Autodesk Inventor part; units mm, degrees
ref_plane "YZ Plane" through (0, 0, 0) normal (1, 0, 0) x (0, 1, 0)
ref_plane "XZ Plane" through (0, 0, 0) normal (0, 1, 0) x (-1, 0, 0)
ref_plane "XY Plane" through (0, 0, 0) normal (0, 0, 1) x (1, 0, 0)
sketch "Эскиз1" plane through (0, 0, 0) normal (0, 0, 1) x (1, 0, 0)
  circle A0 centre (0, 0) radius 13
  circle A1 centre (0, 9) radius 1.5
  circle A2 centre (-9, 0) radius 1.5
  circle A3 centre (0, -9) radius 1.5
  circle A4 centre (9, 0) radius 1.5
  dimension "d0" = 26
  dimension "d1" = 3
  dimension "d2" = 9
  dimension "d5" = 360
extrude "Выдавливание1" add sketch "Эскиз1" along normal blind 7
sketch "Эскиз2" plane through (0, 0, 7) normal (0, 0, 1) x (1, 0, 0)
  circle A0 centre (0, 0) radius 13
  circle A1 centre (9, 0) radius 1.5
  circle A2 centre (0, -9) radius 1.5
  circle A3 centre (-9, 0) radius 1.5
  circle A4 centre (0, 9) radius 1.5
  circle A5 centre (0, 0) radius 9.5
  dimension "d9" = 19
extrude "Выдавливание2" add sketch "Эскиз2" along normal blind 5 contours A0 | A1 A5 | A5 A4 | A2 A5 | A5 A3 picked at (9.8174, -0.2697) picked at (-0.0593, 9.8216) picked at (0.0593, -9.8216) picked at (-9.8216, 0.0593)
sketch "Эскиз3" plane through (0, 0, 7) normal (0, 0, 1) x (1, 0, 0)
  arc A0 (-1.4487, 9.3889) -> (-9.3889, 1.4487) centre (0, 0) ccw
  arc A1 (-9.3889, -1.4487) -> (-9.3889, 1.4487) centre (-9, 0) ccw
  arc A2 (-9.3889, -1.4487) -> (-1.4487, -9.3889) centre (0, 0) ccw
  arc A3 (1.4487, -9.3889) -> (-1.4487, -9.3889) centre (0, -9) ccw
  arc A4 (1.4487, -9.3889) -> (9.3889, -1.4487) centre (0, 0) ccw
  arc A5 (9.3889, 1.4487) -> (9.3889, -1.4487) centre (9, 0) ccw
  arc A6 (9.3889, 1.4487) -> (1.4487, 9.3889) centre (0, 0) ccw
  arc A7 (-1.4487, 9.3889) -> (1.4487, 9.3889) centre (0, 9) ccw
  arc A8 (1.4487, 9.3889) -> (-1.4487, 9.3889) centre (0, 0) ccw
  circle A9 centre (0, 0) radius 9.5
  arc A10 (9.3889, -1.4487) -> (9.3889, 1.4487) centre (0, 0) ccw
  arc A11 (1.4487, -9.3889) -> (9.3889, -1.4487) centre (0, 0) ccw
  arc A12 (-1.4487, -9.3889) -> (1.4487, -9.3889) centre (0, 0) ccw
  arc A13 (-9.3889, -1.4487) -> (-1.4487, -9.3889) centre (0, 0) ccw
  arc A14 (-9.3889, 1.4487) -> (-9.3889, -1.4487) centre (0, 0) ccw
  arc A15 (-1.4487, 9.3889) -> (-9.3889, 1.4487) centre (0, 0) ccw
  arc A16 (1.4487, 9.3889) -> (-1.4487, 9.3889) centre (0, 0) ccw
  arc A17 (9.3889, 1.4487) -> (1.4487, 9.3889) centre (0, 0) ccw
  point P0 (-1.4487, -9.3889)
  point P1 (1.4487, -9.3889)
  point P2 (9.3889, -1.4487)
  point P3 (9.3889, 1.4487)
  point P4 (-9.3889, 1.4487)
  point P5 (-9.3889, -1.4487)
extrude "Выдавливание3" add sketch "Эскиз3" against normal blind 0.1 contours A8 A7 | A1 A9 | A9 A5 | A3 A9
sketch "Эскиз4" plane through (0, 0, 12) normal (0, 0, 1) x (1, 0, 0)
  circle A0 centre (-16.4751, 0) radius 1.5
  circle A1 centre (0, 9) radius 1.5
  arc A2 (1.4487, -9.3889) -> (-1.4487, -9.3889) centre (0, -9) ccw
  line L0 (0, 9) -> (0, -9)
  circle A3 centre (16.4751, 0) radius 1.5
  line L1 (-19.9502, -2.5984) -> (-13, -2.5984)
  line L2 (-13, -2.5984) -> (-13, 2.5984)
  line L3 (-13, 2.5984) -> (-19.9502, 2.5984)
  line L4 (-19.9502, 2.5984) -> (-19.9502, -2.5984)
  line L5 (-19.9502, -2.5984) -> (-13, 2.5984) construction
  line L6 (-13, -2.5984) -> (-19.9502, 2.5984) construction
  line L7 (-13, 2.5984) -> (-11.6906, 2.5984)
  circle A4 centre (0, 0) radius 13
  circle A5 centre (0, 0) radius 9.5
  line L8 (-13, -2.5984) -> (-12.3453, -2.5984)
  circle A6 centre (16.4751, 0) radius 1.5
  line L9 (19.9502, -2.5984) -> (13, -2.5984)
  line L10 (13, -2.5984) -> (13, 2.5984)
  line L11 (13, 2.5984) -> (19.9502, 2.5984)
  line L12 (19.9502, 2.5984) -> (19.9502, -2.5984)
  line L13 (19.9502, -2.5984) -> (13, 2.5984) construction
  line L14 (13, -2.5984) -> (19.9502, 2.5984) construction
  line L15 (13, 2.5984) -> (11.6906, 2.5984)
  line L16 (13, -2.5984) -> (12.3453, -2.5984)
  point P0 (12.7377, 2.5984)
  point P1 (12.7377, -2.5984)
  point P2 (-12.7377, -2.5984)
  point P3 (-12.7377, 2.5984)
  dimension "d14" = 3
extrude "Выдавливание4" add sketch "Эскиз4" against normal blind 3 contours L4 L3 L2 L1 | L2 A4 L8 | L2 L7 A4 | A4 L10 L16 | L15 L10 A4 | L10 L11 L12 L9
properties part number "вт2"
Can you work these out from the model? Positions are in its coordinate system, mm. A direction names the side the tool comes from. Coordinates: 2 decimals unless noted, no trailing zeros. Write each loop counter-clockwise with the first axis right and the second up, starting at its lowest first coordinate (ties: lowest second). Pieces come first, ordered by that corner, then holes. Notation, with made-up numbers: M -8,67 L 3,67 A17 cw 3,78 Z; hole C -27,19.5 d8. An arc over 180 degrees is marked long. Use one line per item in the form item = value.
Q1. For faces 5 (the flat face through (-16, 2.598, 11)), 6 (the flat face through (16, 2.598, 11)), 7 (the flat face through (-10, 0, 7)), which set-ups out of +Z, -Z, +X, -X, +Y, -Y let a thin tool reach every point of the face, with its end or its side?
Model answer:
face_5 = +Z, -Z, -X, +Y
face_6 = +Z, -Z, +X, +Y
face_7 = -Z
Q2. I need wall thicknesses on line 1 along Y through (x, z) = (0, 2); line 2 along Y through (x, z) = (9, 2.5); line 3 along Y through (x, z) = (0, 9). Which ranges of each line are inside material? Lowest first, please. Write a range as from..to.
Model answer:
line_1 = -13..-10.5, -7.5..7.5, 10.5..13
line_2 = -9.38..-1.5, 1.5..9.38
line_3 = -13..-9.5, 9.5..13
Q3. For P1, Ø4, axis at y = 3.5, z = 7, coming from the +X side; P2, Ø0.6, axis at x = 10, y = 0, coming from the -Z side; P3, Ø2, axis at x = 1.5, z = 7, coming from the +Y side, each with a flat end and sliding along its axis, tell me the tip position at first contact or that it passes through.
Model answer:
P1 = 12.91
P2 = 7
P3 = 12.99
Q4. We'd pull the mould along Y, two halves only. Please class faces 1 (the flat face through (0, 10, 7)), 2 (the cylindrical face through (17.906, 0.451, 10.521)), 3 (the flat face through (16, -2.598, 11)), 4 (the flat face through (0, -10, 12)): +Y half, -Y half, draft (parallel to the pull), parting line (faces both ways), or undercut.
Model answer:
face_1 = undercut
face_2 = undercut
face_3 = -Y half
face_4 = draft
Q5. If we section it at B-B (z = 3): Write out the boundary of the cut face in (x, y).
Model answer:
outline = C 0,0 d26; hole C -9,0 d3; hole C 0,-9 d3; hole C 0,9 d3; hole C 9,0 d3
Q6. If we section it at D-D (z = 7.75): Write out the boundary of the cut face in (x, y).
Model answer:
outline = C 0,0 d26; hole C 0,0 d19
